Design review of the part built by this model. Coordinates are the model's own, in mm. A direction names the side the tool comes from. Give positions to 0.01 mm unless a question says otherwise; leave off trailing zeros. Order: outer loops, then holes, each group sorted by start corner. A loop starts at its lowest first (then second) coordinate and runs counter-clockwise, first axis right, second up. Notation, with made-up numbers: M -10,55 L 25,55 A9 cw 25,69 Z; hole C 3,78.5 d4. An arc over 180 degrees is marked long. Answer as a JSON object with one key per item and string values.
from build123d import *

# Parameters (mm, degrees)
ESQUISSE1_W        = 12
ESQUISSE1_H        = 12
ESQUISSE1_W_2      = 6
ESQUISSE1_H_2      = 6
BOSS_EXTRU_1_DEPTH = 20
ESQUISSE2_R        = 2


with BuildPart() as part:
    # Esquisse1 → Boss.-Extru.1 (new, symmetric)
    with BuildSketch(Plane.XY):
        Rectangle(ESQUISSE1_W, ESQUISSE1_H)
        Rectangle(ESQUISSE1_W_2, ESQUISSE1_H_2, mode=Mode.SUBTRACT)
    extrude(amount=BOSS_EXTRU_1_DEPTH, both=True)

    # Balayage1: sweep along a curve in space
    with BuildLine() as balayage1_path:
        Line((0, 6, 0), (0, 9, 0))
        Line((0, 9, 0), (-35, 9, 0))
    # Esquisse2 → Balayage1 (sweep)
    with BuildSketch(Plane(origin=(0, 6, 0), x_dir=(1, 0, 0), z_dir=(0, 1, 0))):
        Circle(ESQUISSE2_R)
    balayage1 = sweep(path=balayage1_path.line, transition=Transition.RIGHT)

    # Esquisse3 → Révolution1 (revolve)
    with BuildSketch(Plane.XY):
        with BuildLine():
            Line((-35, 15.35), (-35, 2.65))
            ThreePointArc((-35, 2.65), (-41.35, 9), (-35, 15.35))
        make_face()
    r_volution1 = revolve(axis=Axis((-35, 15.35, 0), (0, -1, 0)))

    # Symétrie1: Balayage1, Révolution1 across plane
    add(balayage1.mirror(Plane(origin=(0, 0, 0), x_dir=(0, 0, 1), z_dir=(1, 0, 0))))
    add(r_volution1.mirror(Plane(origin=(0, 0, 0), x_dir=(0, 0, 1), z_dir=(1, 0, 0))))


solid = part.part
(1) We need section C-C (z = 10). Write out the cut boundary in (x, y).
Checked values:
{"outline": "M -6,-6 L 6,-6 L 6,6 L -6,6 Z; hole M -3,-3 L 3,-3 L 3,3 L -3,3 Z"}
(2) We need section B-B (z = -3.5). Write out the cut boundary in (x, y).
Checked values:
{"outline": "C -35,9 d10.6; M -6,-6 L 6,-6 L 6,6 L -6,6 Z; C 35,9 d10.6; hole M -3,-3 L 3,-3 L 3,3 L -3,3 Z"}
(3) Insertion check: pin 1 (5 mm diameter, centred on y = 0, z = -9, fed in from -X); pin 2 (12 mm diameter, centred on x = -7, y = 9, fed in from +Z); pin 3 (3.5 mm diameter, centred on x = 2, z = 4, fed in from +Y); pin 4 (5 mm diameter, centred on y = -1, z = 6, fed in from +X). Each pin has a flat end and moves straight along its axis. Give the tip position at first contact, or say it passes through.
Checked values:
{"pin 1": "stops at x = -6", "pin 2": "stops at z = 20", "pin 3": "stops at y = 6", "pin 4": "stops at x = 6"}
(4) We need section D-D (z = 5.5). Write out the cut boundary in (x, y), plus the area to 3 significant figures.
Checked values:
{"outline": "C -35,9 d6.35; M -6,-6 L 6,-6 L 6,6 L -6,6 Z; C 35,9 d6.35; hole M -3,-3 L 3,-3 L 3,3 L -3,3 Z", "area": "171 mm^2"}
(5) To check wall thickness, follow L1, parallel to X at y = 7, z = -1; L2, parallel to X at y = 2, z = 14.5; L3, parallel to X at y = 5.75, z = 0. State the ranges of each line that lie inside material, in increasing order. Write a range as from..to.
Checked values:
{"L1": "x = -40.94..-29.06, -1.73..1.73, 29.06..40.94", "L2": "x = -6..-3, 3..6", "L3": "x = -40.46..-29.54, -6..6, 29.54..40.46"}
(6) Draft analysis for pull direction Y (two halves, no side actions). For faces 4 (the flat face through (0, 3, 0)), 5 (the flat face through (0, -6, 0)), 6 (the flat face through (-4, 0, -20)), state which applies: +Y half, -Y half, draft (parallel to the pull), parting line (faces both ways), or undercut.
Checked values:
{"face 4": "undercut", "face 5": "-Y half", "face 6": "draft"}
(7) Tool access review of faces 1 (the cylindrical face through (-1.474, 6.854, -1.352)), 2 (the flat face through (-3, 0, 0)), 3 (the flat face through (-4, 0, 20)): name each direction out of +Z, -Z, +X, -X, +Y, -Y from which nothing blocks a thin tool from reaching the whole face with its end or side.
Checked values:
{"face 1": "none", "face 2": "+Z, -Z", "face 3": "+Z, +X, -X, +Y, -Y"}
(8) We need section A-A (y = -0.25). Write out the cut boundary in (x, z), plus the area to 3 significant figures.
Checked values:
{"outline": "M -6,-20 L -3,-20 L -3,20 L -6,20 Z; M 3,-20 L 6,-20 L 6,20 L 3,20 Z", "area": "240 mm^2"}
